from build123d import *

# Parameters (mm, degrees)
SKETCH1_R           = 1.5
BOSS_EXTRUDE1_DEPTH = 3
FILLET1_R           = 3
SCALE1_SCALE        = 1.9


with BuildPart() as part:
    # Sketch1 → Boss-Extrude1 (new body)
    with BuildSketch(Plane.XY):
        with BuildLine():
            Line((2.948464825, 1.901558102), (27.398838387, 5.123947068))
            ThreePointArc((27.398838387, 5.123947068), (34.199993873, 4.507321028), (27.790827839, 2.149666606))
            Line((27.790827839, 2.149666606), (3.336427979, -1.073252998))
            ThreePointArc((3.336427979, -1.073252998), (-3.463886078, -0.447419324), (2.948464825, 1.901558102))
        make_face()
        Circle(SKETCH1_R, mode=Mode.SUBTRACT)
        with Locations((30.73, 4.05)):
            Circle(SKETCH1_R, mode=Mode.SUBTRACT)
    extrude(amount=-BOSS_EXTRUDE1_DEPTH)

    # Fillet1
    fillet1_edges = [part.edges().sort_by_distance(p)[0] for p in [
        (3.336427979, -1.073252998, -1.5),
        (2.948464825, 1.901558102, -1.5),
        (27.398838387, 5.123947068, -1.5),
        (27.790827839, 2.149666606, -1.5),
    ]]
    fillet(fillet1_edges, radius=FILLET1_R)


with BuildPart() as part_1:
    # Scale1: scaled about (15.368858916, 2.026731994, -1.5)
    add(part.part.scale(SCALE1_SCALE).moved(Location((-13.831973024, -1.824058795, 1.35))))


solid = part_1.part
The model under review builds one solid part; all positions refer to its coordinate system, in mm. A direction names the side the tool comes from. Round coordinates to 2 decimals unless told otherwise and drop trailing zeros. Write each loop counter-clockwise with the first axis right and the second up, starting at its lowest first coordinate (ties: lowest second). Pieces come first, ordered by that corner, then holes. Notation, with made-up numbers: M 82,37.25 L 105,37.25 A11 cw 105,43.25 Z; hole C 16,-20 d8. An arc over 180 degrees is marked long. Use a Markdown table: item, result. Add a question column.
Q1. The part is to be moulded in two halves that separate along Y. For faces 1 (the face through (47.273, 6.727, -1.46)), 2 (the face through (-7.595, 2.322, -1.54)), 3 (the face through (51.115, 6.959, -1.46)), say which applies: pulls with the +Y half, pulls with the -Y half, needs draft (parallel to the pull), parting line crosses it, or undercut.
Q2. To check wall thickness, follow line 1 (X direction, y = -4, z = -2.7); line 2 (Y direction, x = -17, z = -0.2); line 3 (Y direction, x = 37.5, z = -0.75). State the ranges of each line that lie inside material, in increasing order.
Q3. Insertion check: pin 1 (2 mm diameter, centred on x = 40.5, z = -1, fed in from +Y); pin 2 (1.5 mm diameter, centred on x = 25, y = 8.5, fed in from -Z); pin 3 (3 mm diameter, centred on x = -6.5, z = -1, fed in from +Y). Each pin has a flat end and moves straight along its axis. Give the tip position at first contact, or say it passes through.
Q4. We need section B-B, the plane z = -3.45. State the section outline as (x, y) points.
Q5. We need section C-C, the plane x = 20.5. State the section outline as (y, z) points.
Q6. Machinability: for faces 4 (the face through (16.022, -0.764, -1.46)), 5 (the face through (-16.68, -1.7, -1.46)), 6 (the face through (14.715, 4.813, -1.46)), which of the approach directions +Z, -Z, +X, -X, +Y, -Y give a long, thin tool a straight path to every point of the face, cutting with its end or side? Answer none if there is none.
Q7. We need section A-A, the plane x = 44.5. State the section outline as (y, z) points, plus the area to 3 significant figures.
Findings below:
| question | item | result |
|---|---|---|
| 1 | face 1 | undercut |
| 1 | face 2 | pulls with the +Y half |
| 1 | face 3 | parting line crosses it |
| 2 | line 1 | x = -20.1 to -15.67, -11.99 to -6.35 |
| 2 | line 2 | y = -7.65 to 4.03 |
| 2 | line 3 | y = 1.89 to 8.27 |
| 3 | pin 1 | stops at y = 11.78 |
| 3 | pin 2 | passes through |
| 3 | pin 3 | stops at y = 2.45 |
| 4 | outline | M -9.66,3.37 A6.65 ccw long -8.46,-5.76 A5.7 cw -4.62,-3.48 L 36.09,1.88 A5.7 cw 40.4,0.68 A6.65 ccw long 39.2,9.81 A5.7 cw 35.35,7.53 L -5.35,2.17 A5.7 cw Z; hole C -13.83,-1.82 d5.7; hole C 44.56,5.87 d5.7 |
| 5 | outline | M -0.17,-4.35 L 5.58,-4.35 L 5.58,1.35 L -0.17,1.35 Z |
| 6 | face 4 | +Z, -Z, -Y |
| 6 | face 5 | +Z, -Z |
| 6 | face 6 | +Z, -Z, +Y |
| 7 | outline | M -0.78,-4.35 L 3.02,-4.35 L 3.02,1.35 L -0.78,1.35 Z; M 8.72,-4.35 L 12.52,-4.35 L 12.52,1.35 L 8.72,1.35 Z |
| 7 | area | 43.3 mm² |
